```python
from build123d import *

# Parameters (mm, degrees)
SKETCH1_W          = 33.02
SKETCH1_H          = 55
BASE_DEPTH         = 3.175
SKETCH3_W          = 39.37
SKETCH3_H          = 61.35
SKETCH3_W_2        = 33.02
SKETCH3_H_2        = 55
OUTER_CASING_DEPTH = 19.05
FILLET1_R          = 1.5875
SKETCH5_R          = 1.143
CUT_EXTRUDE5_DEPTH = 6.35


with BuildPart() as part:
    # Sketch1 → Base (new body)
    with BuildSketch(Plane(origin=(0, 0, 0), x_dir=(1, 0, 0), z_dir=(0, 1, 0))):
        Rectangle(SKETCH1_W, SKETCH1_H)
        Polygon((-16.51, 27.5), (16.51, 27.5), (16.51, -27.5), align=None)
    extrude(amount=BASE_DEPTH)

    # Sketch3 → Outer-Casing (add)
    with BuildSketch(Plane.XZ):
        Rectangle(SKETCH3_W, SKETCH3_H)
        Rectangle(SKETCH3_W_2, SKETCH3_H_2, mode=Mode.SUBTRACT)
    extrude(amount=-OUTER_CASING_DEPTH)

    # Fillet1
    fillet1_edges = [part.edges().sort_by_distance(p)[0] for p in [
        (19.685, 9.525, 30.675),
        (19.685, 9.525, -30.675),
        (-19.685, 9.525, -30.675),
        (-19.685, 9.525, 30.675),
        (19.685, 0, 0),
        (0, 0, 30.675),
        (-19.685, 0, 0),
        (0, 0, -30.675),
    ]]
    fillet(fillet1_edges, radius=FILLET1_R)

    # Sketch5 → Cut-Extrude5 (cut)
    with BuildSketch(Plane(origin=(0, 19.05, 0), x_dir=(1, 0, 0), z_dir=(0, 1, 0))):
        with Locations(Location((-17.767235857, 28.757235857, 0), (0, 0, 270))):
            Circle(SKETCH5_R)
        with Locations(Location((-17.767235857, -28.757235857, 0), (0, 0, 270))):
            Circle(SKETCH5_R)
        with Locations(Location((17.767235857, -28.757235857, 0), (0, 0, 270))):
            Circle(SKETCH5_R)
        with Locations(Location((17.767235857, 28.757235857, 0), (0, 0, 270))):
            Circle(SKETCH5_R)
    extrude(amount=-CUT_EXTRUDE5_DEPTH, mode=Mode.SUBTRACT)


solid = part.part
```
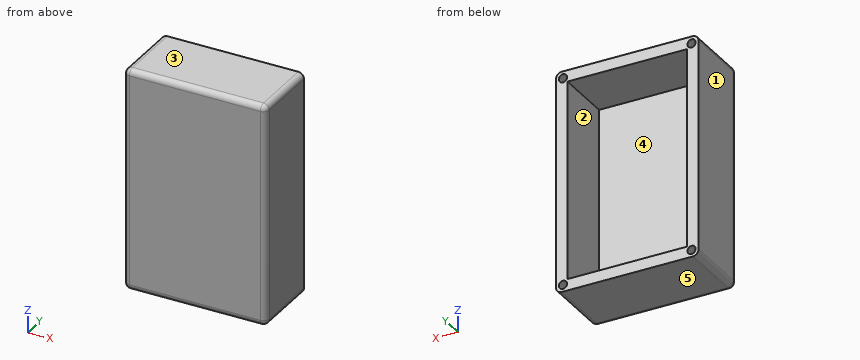
Model file for the job. Use its own axes, mm. Face numbers are marked on the shaded views. A direction names the side the tool comes from. Round coordinates to 2 decimals unless told otherwise and drop trailing zeros. Write each loop counter-clockwise with the first axis right and the second up, starting at its lowest first coordinate (ties: lowest second). Pieces come first, ordered by that corner, then holes. Notation, with made-up numbers: (-21.5, -2) - (-9.5, -2) arc R30 cw to (-9.5, 20) - close; hole circle Ø6 at (71.5, 41). An arc over 180 degrees is marked (long way). One line per item, written item: value.
(1) 3-axis set-ups, long thin cutter, end or side, ignore diameter. For the marked faces 4 and 5: which of +Z, -Z, +X, -X, +Y, -Y reach the whole face in a straight line?
Values follow:
face 4: +Y
face 5: -Z, +X, -X, +Y, -Y
(2) Wall check: probe 1 along Z at (x, y) = (12.5, 11.75) (3 decimals); probe 2 along X at (y, z) = (10, -2) (3 decimals); probe 3 along Z at (x, y) = (17.5, 13) (3 decimals). Give the ranges that are in metal, low to high.
Values follow:
probe 1: z = -30.675 to -27.5, 27.5 to 30.675
probe 2: x = -19.685 to -16.51, 16.51 to 19.685
probe 3: z = -30.675 to -29.869, -27.646 to 27.646, 29.869 to 30.675
(3) Cut at A-A, the plane y = 4. Give the cut face in (x, z) (1 decimal).
Values follow:
outline: (-19.7, -29.1) arc R1.6 ccw to (-18.1, -30.7) - (18.1, -30.7) arc R1.6 ccw to (19.7, -29.1) - (19.7, 29.1) arc R1.6 ccw to (18.1, 30.7) - (-18.1, 30.7) arc R1.6 ccw to (-19.7, 29.1) - close; hole (-16.5, -27.5) - (16.5, -27.5) - (16.5, 27.5) - (-16.5, 27.5) - close
(4) Two-plate mould, pull along X, no slides. Class the marked faces 1, 2 and 3: pulls with the +X half, pulls with the -X half, needs draft (parallel to the pull), parting line crosses it, or undercut.
Values follow:
face 1: pulls with the -X half
face 2: undercut
face 3: needs draft
